Print and shaded views of the part. All mm, measured from the part's lowest x, y and z. A direction names the side the tool comes from. Coordinates: 2 decimals unless noted, no trailing zeros. Order: outer loops, then holes, each group sorted by start corner. A loop starts at its lowest first (then second) coordinate and runs counter-clockwise, first axis right, second up. Notation, with made-up numbers: (-17, 33.5) -> (35, 33.5) arc R23 ccw to (35, 61.5) -> close; hole circle Ø8 at (-2.75, -39). An arc over 180 degrees is marked (long way). Return JSON: item names as keys, results as strings. Group by question number.
1) Cut at C-C (y = 22.5). Write the cut outline in (x, z) (1 decimal).
2) Cut at D-D (z = 36). Write the cut outline in (x, y) (1 decimal).
3) Cut at A-A (z = 30.5). Write the cut outline in (x, y).
4) Probe line 1 (Y direction, x = 11, z = 28); line 2 (X direction, y = 7.5, z = 20) (1 decimal); line 3 (Z direction, x = 29, y = 24). List the from-to ranges inside material, lowest first.
5) Which spindle directions (+Z, -Z, +X, -X, +Y, -Y) get a long thin tool onto all of the face, cutting with end or side? Do the marked faces 1 and 2. Say none if no direction does.
6) Pull direction Z, two halves, no side cores. Call the marked faces 3, 4 and 5: +Z half, -Z half, draft (parallel to the pull), parting line (faces both ways), or undercut.
7) Cut at B-B (x = 33.5). Write the cut outline in (y, z) (1 decimal).
8) Flat gauge pins, fed straight in: pin 1 (10 mm diameter, centred on y = 23.5, z = 36.5, fed in from -X); pin 2 (8 mm diameter, centred on x = 26.5, y = 24.5, fed in from -Z); pin 3 (3 mm diameter, centred on y = 13, z = 26.5, fed in from -X) (1 decimal). Where does each tip first touch, or does it go through?
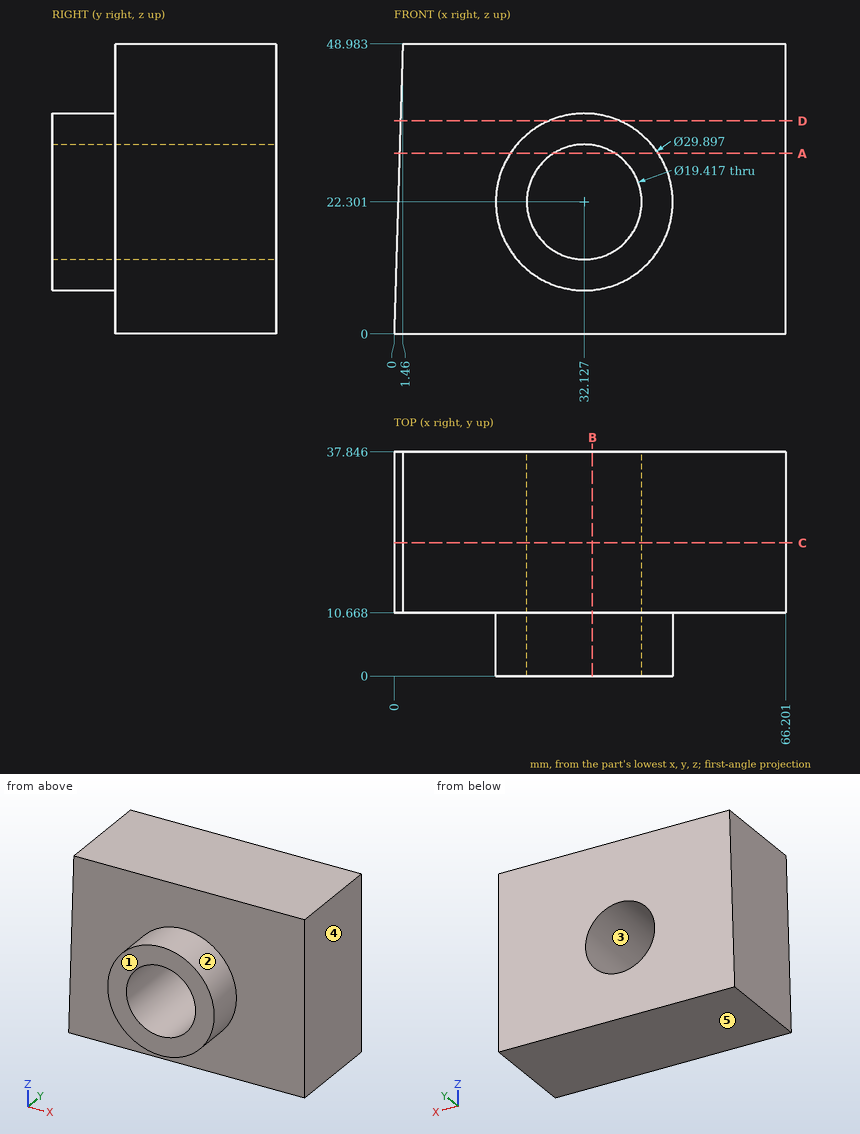
Answers below:
{
 "1": {"outline": "(0, 0) -> (66.2, 0) -> (66.2, 49) -> (1.5, 49) -> close; hole circle Ø19.4 at (32.1, 22.3)"},
 "2": {"outline": "(1.1, 10.7) -> (26.1, 10.7) -> (26.1, 0) -> (38.1, 0) -> (38.1, 10.7) -> (66.2, 10.7) -> (66.2, 37.8) -> (1.1, 37.8) -> close"},
 "3": {"outline": "(0.91, 10.67) -> (19.63, 10.67) -> (19.63, 0) -> (26.93, 0) -> (26.93, 37.85) -> (0.91, 37.85) -> close; (37.33, 0) -> (44.63, 0) -> (44.63, 10.67) -> (66.2, 10.67) -> (66.2, 37.85) -> (37.33, 37.85) -> close"},
 "4": {"line 1": "y = 10.67 to 37.85", "line 2": "x = 17.4 to 22.7, 41.6 to 46.9", "line 3": "z = 0 to 13.11, 31.49 to 48.98"},
 "5": {"face 1": "+Z, -Z, +X, -X, -Y", "face 2": "-Y"},
 "6": {"face 3": "undercut", "face 4": "draft", "face 5": "-Z half"},
 "7": {"outline": "(0, 7.4) -> (10.7, 7.4) -> (10.7, 0) -> (37.8, 0) -> (37.8, 12.7) -> (0, 12.7) -> close; (0, 31.9) -> (37.8, 31.9) -> (37.8, 49) -> (10.7, 49) -> (10.7, 37.2) -> (0, 37.2) -> close"},
 "8": {"pin 1": "stops at x = 0.94", "pin 2": "stops at z = 0", "pin 3": "stops at x = 0.7"}
}
